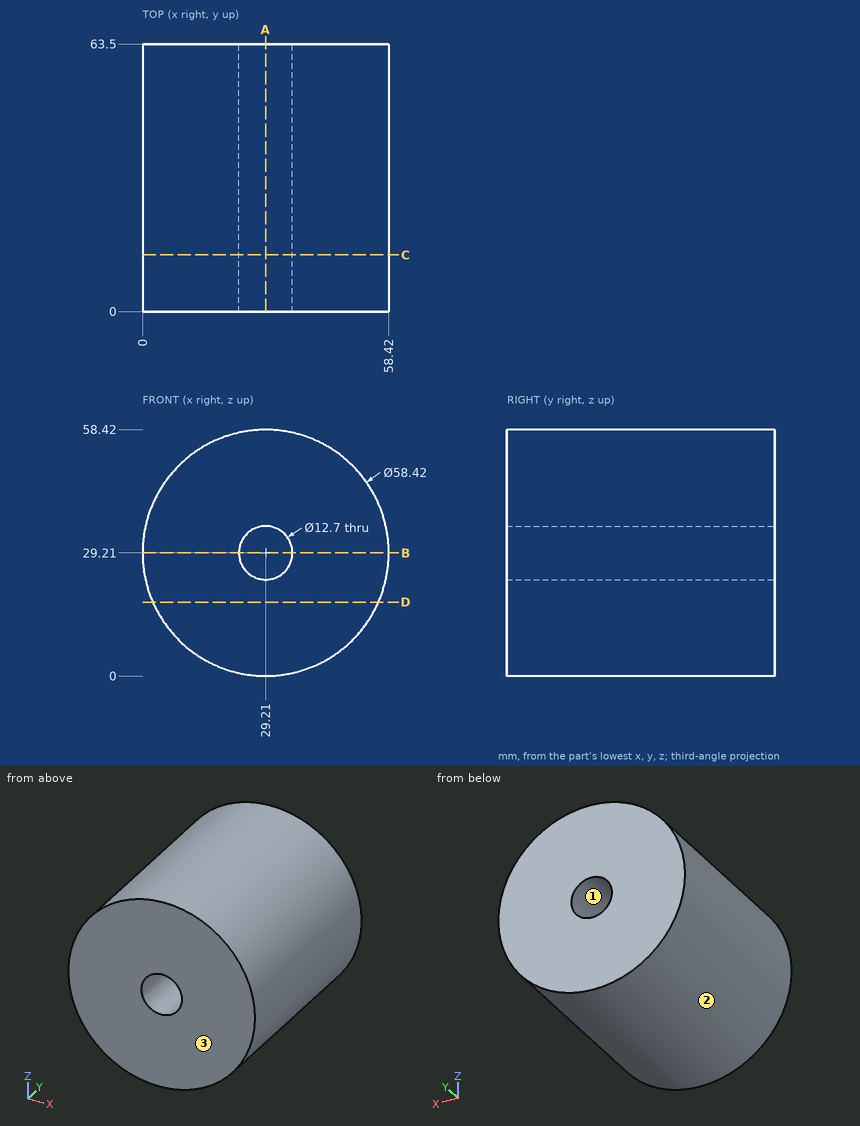
Drawing for the job (mm, zero at the part's lowest x, y, z). Coordinates: 2 decimals unless noted, no trailing zeros. Order: outer loops, then holes, each group sorted by start corner. A loop starts at its lowest first (then second) coordinate and runs counter-clockwise, first axis right, second up.
Item 1: Pin check, flat tips, straight feed: pin 1 Ø5 at (x, y) = (23.5, 43.5) entering from +Z; pin 2 Ø1.5 at (x, y) = (29, 22) entering from +Z; pin 3 Ø8 at (x, y) = (26.5, 35) entering from -Z. Stop position of each tip, or through.
Check sheet entries:
pin 1: stops at z = 58.24
pin 2: stops at z = 58.42
pin 3: stops at z = 0
Item 2: Band-saw the part on C-C on y = 13.5. List the corners of the cut face in (x, z), plus the area to 3 significant figures.
Check sheet entries:
outline: circle Ø58.42 at (29.21, 29.21); hole circle Ø12.7 at (29.21, 29.21)
area: 2,550 mm2
Item 3: Band-saw the part on D-D on z = 17.5. List the corners of the cut face in (x, y).
Check sheet entries:
outline: (2.45, 0) - (55.97, 0) - (55.97, 63.5) - (2.45, 63.5) - close
Item 4: Band-saw the part on B-B on z = 29.21. List the corners of the cut face in (x, y), plus the area to 3 significant figures.
Check sheet entries:
outline: (0, 0) - (22.86, 0) - (22.86, 63.5) - (0, 63.5) - close; (35.56, 0) - (58.42, 0) - (58.42, 63.5) - (35.56, 63.5) - close
area: 2,900 mm2
Item 5: Two-plate mould, pull along X, no slides. Class the marked faces 1, 2 and 3: +X half, -X half, draft (parallel to the pull), parting line (faces both ways), or undercut.
Check sheet entries:
face 1: undercut
face 2: parting line
face 3: draft
Item 6: Drill centre lines: L1, parallel to X at y = 45, z = 29; L2, parallel to Z at x = 27, y = 48. Where is each one in solid material? Low to high.
Check sheet entries:
L1: x = 0 to 22.86, 35.56 to 58.42
L2: z = 0.08 to 23.26, 35.16 to 58.34
Item 7: Band-saw the part on A-A on x = 29.21. List the corners of the cut face in (y, z), plus the area to 3 significant figures.
Check sheet entries:
outline: (0, 0) - (63.5, 0) - (63.5, 22.86) - (0, 22.86) - close; (0, 35.56) - (63.5, 35.56) - (63.5, 58.42) - (0, 58.42) - close
area: 2,900 mm2
